For this review, take the finished solid that the model builds, in its own axes (mm). Give positions to 0.01 mm unless a question says otherwise; leave off trailing zeros. Order: outer loops, then holes, each group sorted by start corner. A loop starts at its lowest first (then second) coordinate and runs counter-clockwise, first axis right, second up. Notation, with made-up numbers: (75, 85.25) -> (132, 85.25) arc R7 ccw to (132, 91.25) -> close; hole circle Ø11 at (39, 33). An arc over 180 degrees is marked (long way). Return JSON: item names as keys, results as strings. Group by question number.
1) Insertion check: P1, Ø7, axis at x = 39, z = -80, coming from the -Y side; P2, Ø1.5, axis at x = -176.5, y = 1.5, coming from the -Z side; P3, Ø1.5, axis at y = 1, z = 166.5, coming from the +X side. Each pin has a flat end and moves straight along its axis. Give the tip position at first contact, or say it passes through.
2) Add section B-B (x = -177.5). Give the boundary of the cut face in (y, z), then the cut area to 3 significant figures.
3) Add section A-A (y = 1.6). State how many separate pieces and enclosed holes the cut face has, then the cut area to 3 significant figures.
4) To check wall thickness, follow line 1 along X through (y, z) = (2, 210) (3 decimals); line 2 along Z through (x, y) = (-260, 0.9) (3 decimals); line 3 along Z through (x, y) = (232, 0.85) (3 decimals). State the ranges of each line that lie inside material, in increasing order.
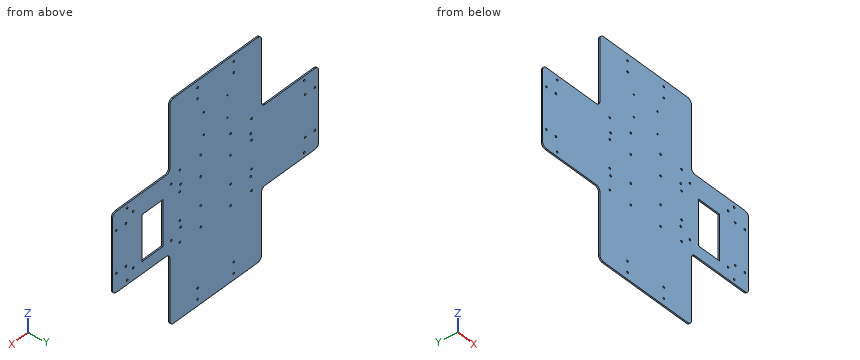
from build123d import *

# Parameters (mm, degrees)
BASE_DEPTH               = 3
FILLET1_R                = 10
SKETCH2_R                = 2.125
ARMOR_MODULE_HOLES_DEPTH = 3
SKETCH3_R                = 2.125
PLATES_FOR_GIMBAL_DEPTH  = 3
SKETCH6_R                = 2.125
SKETCH6_W                = 55
SKETCH6_H                = 104
BATTERY_MOUNT_DEPTH      = 10
SKETCH5_R                = 2.125
SUSPENSION_MOUNT_DEPTH   = 10
SKETCH7_R                = 2.125
OUTER_BOARD_MOUNT_DEPTH  = 10
SKETCH8_R                = 1.575
RFID_DEPTH               = 10


with BuildPart() as part:
    # Sketch1 → Base (new body)
    with BuildSketch(Plane(origin=(0, 0, 0), x_dir=(1, 0, 0), z_dir=(0, 1, 0))):
        Polygon((120, 250), (-120, 250), (-120, 90), (-270, 90), (-270, -90), (-120, -90), (-120, -250), (120, -250), (120, -90), (270, -90), (270, 90), (120, 90), align=None)
    extrude(amount=BASE_DEPTH)

    # Fillet1
    fillet1_edges = [part.edges().sort_by_distance(p)[0] for p in [
        (-270, 1.5, 90),
        (-270, 1.5, -90),
        (-120, 1.5, -90),
        (-120, 1.5, -250),
        (120, 1.5, -250),
        (120, 1.5, -90),
        (270, 1.5, -90),
        (270, 1.5, 90),
        (120, 1.5, 90),
        (120, 1.5, 250),
        (-120, 1.5, 250),
        (-120, 1.5, 90),
    ]]
    fillet(fillet1_edges, radius=FILLET1_R)

    # Sketch2 → Armor Module Holes (cut)
    with BuildSketch(Plane(origin=(0, 3, 0), x_dir=(1, 0, 0), z_dir=(0, 1, 0))):
        with Locations(Location((-47.5, 235, 0), (0, 0, 270))):
            Circle(SKETCH2_R)
        with Locations(Location((-47.5, 210, 0), (0, 0, 270))):
            Circle(SKETCH2_R)
        with Locations(Location((-260, 47.5, 0), (0, 0, 270))):
            Circle(SKETCH2_R)
        with Locations(Location((-235, 47.5, 0), (0, 0, 270))):
            Circle(SKETCH2_R)
        with Locations(Location((-235, -47.5, 0), (0, 0, 90))):
            Circle(SKETCH2_R)
        with Locations(Location((-260, -47.5, 0), (0, 0, 90))):
            Circle(SKETCH2_R)
        with Locations(Location((260, -47.5, 0), (0, 0, 270))):
            Circle(SKETCH2_R)
        with Locations(Location((235, -47.5, 0), (0, 0, 270))):
            Circle(SKETCH2_R)
        with Locations(Location((235, 47.5, 0), (0, 0, 90))):
            Circle(SKETCH2_R)
        with Locations(Location((260, 47.5, 0), (0, 0, 90))):
            Circle(SKETCH2_R)
        with Locations(Location((47.5, 210, 0), (0, 0, 90))):
            Circle(SKETCH2_R)
        with Locations(Location((47.5, 235, 0), (0, 0, 90))):
            Circle(SKETCH2_R)
        with Locations(Location((47.5, -235, 0), (0, 0, 270))):
            Circle(SKETCH2_R)
        with Locations(Location((47.5, -210, 0), (0, 0, 270))):
            Circle(SKETCH2_R)
        with Locations(Location((-47.5, -210, 0), (0, 0, 90))):
            Circle(SKETCH2_R)
        with Locations(Location((-47.5, -235, 0), (0, 0, 90))):
            Circle(SKETCH2_R)
    extrude(amount=-ARMOR_MODULE_HOLES_DEPTH, mode=Mode.SUBTRACT)

    # Sketch3 → Plates for Gimbal (cut)
    with BuildSketch(Plane(origin=(0, 3, 0), x_dir=(1, 0, 0), z_dir=(0, 1, 0))):
        with Locations(Location((92, 47.5, 0), (0, 0, 270))):
            Circle(SKETCH3_R)
        with Locations(Location((92, -47.5, 0), (0, 0, 90))):
            Circle(SKETCH3_R)
        with Locations(Location((-92, -47.5, 0), (0, 0, 270))):
            Circle(SKETCH3_R)
        with Locations(Location((-92, 47.5, 0), (0, 0, 90))):
            Circle(SKETCH3_R)
    extrude(amount=-PLATES_FOR_GIMBAL_DEPTH, mode=Mode.SUBTRACT)

    # Sketch6 → Battery Mount (cut)
    with BuildSketch(Plane(origin=(0, 3, 0), x_dir=(1, 0, 0), z_dir=(0, 1, 0))):
        with Locations(Location((116, -62.5, 0), (0, 0, 270))):
            Circle(SKETCH6_R)
        with Locations(Location((216, -62.5, 0), (0, 0, 270))):
            Circle(SKETCH6_R)
        with Locations(Location((216, 62.5, 0), (0, 0, 270))):
            Circle(SKETCH6_R)
        with Locations(Location((116, 62.5, 0), (0, 0, 270))):
            Circle(SKETCH6_R)
        with Locations((166, 10.5)):
            Rectangle(SKETCH6_W, SKETCH6_H)
    extrude(amount=-BATTERY_MOUNT_DEPTH, mode=Mode.SUBTRACT)

    # Sketch5 → Suspension Mount (cut)
    with BuildSketch(Plane(origin=(0, 3, 0), x_dir=(1, 0, 0), z_dir=(0, 1, 0))):
        with Locations(Location((94, -32, 0), (0, 0, 270))):
            Circle(SKETCH5_R)
        with Locations(Location((94, -80, 0), (0, 0, 270))):
            Circle(SKETCH5_R)
        with Locations(Location((39, -32, 0), (0, 0, 270))):
            Circle(SKETCH5_R)
        with Locations(Location((39, -80, 0), (0, 0, 270))):
            Circle(SKETCH5_R)
        with Locations(Location((-39, -80, 0), (0, 0, 270))):
            Circle(SKETCH5_R)
        with Locations(Location((-39, -32, 0), (0, 0, 270))):
            Circle(SKETCH5_R)
        with Locations(Location((-94, -80, 0), (0, 0, 270))):
            Circle(SKETCH5_R)
        with Locations(Location((-94, -32, 0), (0, 0, 270))):
            Circle(SKETCH5_R)
        with Locations(Location((-94, 32, 0), (0, 0, 270))):
            Circle(SKETCH5_R)
        with Locations(Location((-94, 80, 0), (0, 0, 270))):
            Circle(SKETCH5_R)
        with Locations(Location((-39, 32, 0), (0, 0, 270))):
            Circle(SKETCH5_R)
        with Locations(Location((-39, 80, 0), (0, 0, 270))):
            Circle(SKETCH5_R)
        with Locations(Location((39, 80, 0), (0, 0, 270))):
            Circle(SKETCH5_R)
        with Locations(Location((39, 32, 0), (0, 0, 270))):
            Circle(SKETCH5_R)
        with Locations(Location((94, 80, 0), (0, 0, 270))):
            Circle(SKETCH5_R)
        with Locations(Location((94, 32, 0), (0, 0, 270))):
            Circle(SKETCH5_R)
    extrude(amount=-SUSPENSION_MOUNT_DEPTH, mode=Mode.SUBTRACT)

    # Sketch7 → Outer Board Mount (cut)
    with BuildSketch(Plane(origin=(0, 3, 0), x_dir=(1, 0, 0), z_dir=(0, 1, 0))):
        with Locations(Location((-232, -80, 0), (0, 0, 270))):
            Circle(SKETCH7_R)
        with Locations(Location((-232, 80, 0), (0, 0, 270))):
            Circle(SKETCH7_R)
        with Locations(Location((232, 80, 0), (0, 0, 270))):
            Circle(SKETCH7_R)
        with Locations(Location((232, -80, 0), (0, 0, 270))):
            Circle(SKETCH7_R)
    extrude(amount=-OUTER_BOARD_MOUNT_DEPTH, mode=Mode.SUBTRACT)

    # Sketch8 → RFID (cut)
    with BuildSketch(Plane(origin=(0, 3, 0), x_dir=(1, 0, 0), z_dir=(0, 1, 0))):
        with Locations(Location((-31, -120, 0), (0, 0, 270))):
            Circle(SKETCH8_R)
        with Locations(Location((-31, -170, 0), (0, 0, 270))):
            Circle(SKETCH8_R)
        with Locations(Location((31, -170, 0), (0, 0, 270))):
            Circle(SKETCH8_R)
        with Locations(Location((31, -120, 0), (0, 0, 270))):
            Circle(SKETCH8_R)
    extrude(amount=-RFID_DEPTH, mode=Mode.SUBTRACT)


solid = part.part
Evaluation:
{
 "1": {"P1": "y = 0", "P2": "z = -90", "P3": "x = 120"},
 "2": {"outline": "(0, -90) -> (3, -90) -> (3, 90) -> (0, 90) -> close", "area": "540 mm^2"},
 "3": {"separate pieces": "1", "enclosed holes": "49", "area": "168,000 mm^2"},
 "4": {"line 1": "-120 to -49.625, -45.375 to 45.375, 49.625 to 120", "line 2": "-90 to -49.625, -45.375 to 45.375, 49.625 to 90", "line 3": "-90 to -82.125, -77.875 to 77.875, 82.125 to 90"}
}
